For this review, take the finished solid that the model builds, in its own axes (mm). A direction names the side the tool comes from. Coordinates: 2 decimals unless noted, no trailing zeros. Loops run counter-clockwise (first coordinate to the right, second up) from the corner with the lowest first, then second, coordinate; pieces in that order, holes last. Notation, with made-up numbers: M 14.25,7.5 L 63.25,7.5 A15 cw 63.25,33.5 Z; hole C 80.25,70.5 d5. An arc over 180 degrees is marked long. Answer as a JSON object with one key per item and string values. Group by question number.
Item 1: Tool access review of faces 4 (the face through (-5.99, -115.38, 7.4)), 5 (the face through (-7, -5, 7)), 6 (the face through (-4.604, -114.044, 7.395)): name each direction out of +Z, -Z, +X, -X, +Y, -Y from which nothing blocks a thin tool from reaching the whole face with its end or side.
Item 2: Add section B-B (z = 8.25). Count the separate pieces of the cut face and the enclosed holes in it, then the cut area to 3 significant figures.
Item 3: Add section C-C (y = -70.5). State the section outline as (x, z) points.
Item 4: Mouldability with a two-part tool opening along Y and no side actions: class faces 1 (the face through (-11, -20, 7)), 2 (the face through (0, -33, 7)), 3 (the face through (-13.81, -118.7, 7.4)) as +Y half, -Y half, draft (parallel to the pull), parting line (faces both ways), or undercut.
Item 5: Add section A-A (y = -43). State the section outline as (x, z) points.
Item 6: Insertion check: pin 1 (7.5 mm diameter, centred on x = -28, z = 11, fed in from +Y); pin 2 (1.8 mm diameter, centred on y = -90.5, z = 11, fed in from +X); pin 3 (11.5 mm diameter, centred on x = -15, y = -105, fed in from +Z); pin 4 (5 mm diameter, centred on y = -7.5, z = 5, fed in from -X). Each pin has a flat end and moves straight along its axis. Give the tip position at first contact, or say it passes through.
Item 7: Wall thickness on L1, parallel to Y at x = -4.5, z = 11.25; L2, parallel to Y at x = -33, z = 12.5; L3, parallel to Y at x = -6.5, z = 6.75: over which ranges is each line inside the solid? List them lowest first. Write a range as from..to.
from build123d import *

# Parameters (mm, degrees)
SKETCH1_R           = 5
BOSS_EXTRUDE1_DEPTH = 15
CUT_EXTRUDE1_START  = -15
CUT_EXTRUDE1_DEPTH  = 15
BOSS_EXTRUDE2_START = -15
BOSS_EXTRUDE2_DEPTH = 15
FILLET1_R           = 10


with BuildPart() as part:
    # Sketch1 → Boss-Extrude1 (new body)
    with BuildSketch(Plane.XY):
        with BuildLine():
            Line((0, 0), (-10, 0))
            Line((-10, 0), (-48.033043506, -60))
            Line((-48.033043506, -60), (-30, -105))
            ThreePointArc((-30, -105), (-1.41305071, -111.355691072), (-24.614025467, -93.486073028))
            Line((-24.614025467, -93.486073028), (-36.029372005, -65))
            Line((-36.029372005, -65), (0, -65))
            Line((0, -65), (0, 0))
        make_face()
        Polygon((-5, -50), (-5, -60), (-43.033043506, -60), (-36.694202922, -50), align=None, mode=Mode.SUBTRACT)
        Polygon((-27.185942045, -35), (-5, -35), (-5, -45), (-33.52478263, -45), align=None, mode=Mode.SUBTRACT)
        Polygon((-17.677681169, -20), (-5, -20), (-5, -30), (-24.016521753, -30), align=None, mode=Mode.SUBTRACT)
        Polygon((-14.508260877, -15), (-8.169420292, -5), (-5, -5), (-5, -15), align=None, mode=Mode.SUBTRACT)
        with Locations((-15, -105)):
            Circle(SKETCH1_R, mode=Mode.SUBTRACT)
    extrude(amount=BOSS_EXTRUDE1_DEPTH)

    # Sketch2 → Cut-Extrude1 (cut)
    with BuildSketch(Plane.XY.offset(15).offset(CUT_EXTRUDE1_START)):
        with BuildLine():
            Line((-15, -90), (-15, -92.5))
            ThreePointArc((-15, -92.5), (-3.506810704, -109.914936399), (-24.038127106, -113.634944031))
            Line((-24.038127106, -113.634944031), (-25.845752528, -115.361932837))
            ThreePointArc((-25.845752528, -115.361932837), (-1.208172845, -110.897923679), (-15, -90))
        make_face()
    extrude(amount=CUT_EXTRUDE1_DEPTH, mode=Mode.SUBTRACT)

    # Sketch3 → Boss-Extrude2 (add)
    with BuildSketch(Plane.XY.offset(15).offset(BOSS_EXTRUDE2_START)):
        with BuildLine():
            ThreePointArc((-10.467166144, -93.116837157), (-11.06981717, -92.904141005), (-11.682391753, -92.721986422))
            Line((-11.682391753, -92.721986422), (-12.122200649, -90.45579864))
            Line((-12.122200649, -90.45579864), (-13.242544435, -90.278353616))
            Line((-13.242544435, -90.278353616), (-14.361118089, -92.29771785))
            ThreePointArc((-14.361118089, -92.29771785), (-14.499431062, -92.291515722), (-14.637803355, -92.286819615))
            ThreePointArc((-14.637803355, -92.286819615), (-14.818883312, -92.282950867), (-15, -92.281661197))
            Line((-15, -92.281661197), (-15, -92.5))
            ThreePointArc((-15, -92.5), (-3.506810704, -109.914936399), (-24.038127106, -113.634944031))
            Line((-24.038127106, -113.634944031), (-24.195997015, -113.785771498))
            ThreePointArc((-24.195997015, -113.785771498), (-23.126415999, -114.783532334), (-21.949347795, -115.651887492))
            Line((-21.949347795, -115.651887492), (-22.231355215, -117.943068572))
            Line((-22.231355215, -117.943068572), (-21.220678485, -118.458034088))
            Line((-21.220678485, -118.458034088), (-19.532833856, -116.883162843))
            ThreePointArc((-19.532833856, -116.883162843), (-18.93018283, -117.095858995), (-18.317608247, -117.278013578))
            Line((-18.317608247, -117.278013578), (-17.877799351, -119.54420136))
            Line((-17.877799351, -119.54420136), (-16.757455565, -119.721646384))
            Line((-16.757455565, -119.721646384), (-15.638881911, -117.70228215))
            ThreePointArc((-15.638881911, -117.70228215), (-15, -117.718338803), (-14.361118089, -117.70228215))
            Line((-14.361118089, -117.70228215), (-13.242544435, -119.721646384))
            Line((-13.242544435, -119.721646384), (-12.12220065, -119.544201361))
            Line((-12.12220065, -119.544201361), (-11.682391753, -117.278013578))
            ThreePointArc((-11.682391753, -117.278013578), (-11.06981717, -117.095858995), (-10.467166144, -116.883162843))
            Line((-10.467166144, -116.883162843), (-8.779321515, -118.458034088))
            Line((-8.779321515, -118.458034088), (-7.768644785, -117.943068573))
            Line((-7.768644785, -117.943068573), (-8.050652205, -115.651887492))
            ThreePointArc((-8.050652205, -115.651887492), (-7.524348018, -115.289352232), (-7.016919559, -114.900836762))
            Line((-7.016919559, -114.900836762), (-4.925021947, -115.877055647))
            Line((-4.925021947, -115.877055647), (-4.122944353, -115.074978053))
            Line((-4.122944353, -115.074978053), (-5.099163238, -112.983080441))
            ThreePointArc((-5.099163238, -112.983080441), (-4.710647768, -112.475651982), (-4.348112508, -111.949347795))
            Line((-4.348112508, -111.949347795), (-2.056931428, -112.231355215))
            Line((-2.056931428, -112.231355215), (-1.541965913, -111.220678485))
            Line((-1.541965913, -111.220678485), (-3.116837157, -109.532833856))
            ThreePointArc((-3.116837157, -109.532833856), (-2.904141005, -108.93018283), (-2.721986422, -108.317608247))
            Line((-2.721986422, -108.317608247), (-0.45579864, -107.877799351))
            Line((-0.45579864, -107.877799351), (-0.278353616, -106.757455565))
            Line((-0.278353616, -106.757455565), (-2.29771785, -105.638881911))
            ThreePointArc((-2.29771785, -105.638881911), (-2.281661197, -105), (-2.29771785, -104.361118089))
            Line((-2.29771785, -104.361118089), (-0.278353616, -103.242544435))
            Line((-0.278353616, -103.242544435), (-0.45579864, -102.122200649))
            Line((-0.45579864, -102.122200649), (-2.721986422, -101.682391753))
            ThreePointArc((-2.721986422, -101.682391753), (-2.904141005, -101.06981717), (-3.116837157, -100.467166144))
            Line((-3.116837157, -100.467166144), (-1.541965912, -98.779321515))
            Line((-1.541965912, -98.779321515), (-2.056931427, -97.768644785))
            Line((-2.056931427, -97.768644785), (-4.348112508, -98.050652205))
            ThreePointArc((-4.348112508, -98.050652205), (-4.710647768, -97.524348018), (-5.099163238, -97.016919559))
            Line((-5.099163238, -97.016919559), (-4.122944353, -94.925021947))
            Line((-4.122944353, -94.925021947), (-4.925021947, -94.122944353))
            Line((-4.925021947, -94.122944353), (-7.016919559, -95.099163238))
            ThreePointArc((-7.016919559, -95.099163238), (-7.524348018, -94.710647768), (-8.050652205, -94.348112508))
            Line((-8.050652205, -94.348112508), (-7.768644785, -92.056931428))
            Line((-7.768644785, -92.056931428), (-8.779321515, -91.541965912))
            Line((-8.779321515, -91.541965912), (-10.467166144, -93.116837157))
        make_face()
    extrude(amount=BOSS_EXTRUDE2_DEPTH)

    # Fillet1
    fillet1_edges = [part.edges().sort_by_distance(p)[0] for p in [
        (-48.033043506, -60, 7.5),
    ]]
    fillet(fillet1_edges, radius=FILLET1_R)


solid = part.part
From the geometry:
{
 "1": {"face 4": "+Z, -Z, -Y", "face 5": "+Z, -Z", "face 6": "+Z, -Z, +X"},
 "2": {"separate pieces": "1", "enclosed holes": "5", "area": "2,030 mm²"},
 "3": {"outline": "M -43.83,0 L -33.83,0 L -33.83,15 L -43.83,15 Z"},
 "4": {"face 1": "undercut", "face 2": "draft", "face 3": "-Y half"},
 "5": {"outline": "M -37.26,0 L -32.26,0 L -32.26,15 L -37.26,15 Z; M -5,0 L 0,0 L 0,15 L -5,15 Z"},
 "6": {"pin 1": "stops at y = -22.48", "pin 2": "stops at x = -11.94", "pin 3": "stops at z = 15", "pin 4": "stops at x = -16.34"},
 "7": {"L1": "y = -115.45..-114.27, -112.18..-97.82, -95.73..-94.55, -65..0", "L2": "y = -97.51..-72.56, -65..-60, -50..-45, -44.17..-36.28", "L3": "y = -115.14..-94.86, -65..-60, -50..-45, -35..-30, -20..-15, -5..0"}
}
